For this review, take the finished solid that the model builds, in its own axes (mm). A direction names the side the tool comes from. Give positions to 0.01 mm unless a question says otherwise; leave off trailing zeros. Order: outer loops, then holes, each group sorted by start corner. A loop starts at its lowest first (then second) coordinate and runs counter-clockwise, first axis right, second up. Notation, with made-up numbers: (44.5, 35) - (103.5, 35) arc R13 cw to (103.5, 45) - close; hole circle Ø9 at (-28, -6.75). An arc over 180 degrees is marked (long way). Use a Markdown table: item, result. Add a question column.
1) Wall thickness on L1, parallel to Z at x = 4.75, y = 10.7; L2, parallel to X at y = 4.25, z = 5; L3, parallel to X at y = 5, z = 21.05: over which ranges is each line inside the solid? List them lowest first.
2) We need section A-A on x = 22.25. Write out the cut boundary in (y, z).
3) We need section D-D on z = 2. Write out the cut boundary in (x, y).
4) Mouldability with a two-part tool opening along Y and no side actions: class faces 1 (the face through (25.55, 8.41, 23.99)), 2 (the face through (2, 2, 25)), 3 (the face through (0.285, 11.699, 11.154)) as released by +Y, released by -Y, zero draft, split by the parting line, or undercut.
5) Clearance check with flat-ended pins moving along their axes: P1, Ø6.5, axis at x = 13.5, y = 5, coming from the -Z side; P2, Ø3.5, axis at x = 14.5, y = 4, coming from the +Z side; P3, Ø5.5, axis at x = 22.25, z = 8.5, coming from the -Y side; P4, Ø4, axis at x = 4.75, z = 8.5, coming from the -Y side. State where each tip first meets the part, or that it passes through.
6) We need section C-C on y = 5. Write out the cut boundary in (x, z), then the cut area to 3 significant figures.
7) We need section B-B on z = 8.5. Write out the cut boundary in (x, y).
8) Machinability: for faces 4 (the face through (25.25, 5, 10)), 5 (the face through (3.45, 8.48, 23.99)), 6 (the face through (23.55, 1.49, 23.99)), which of the approach directions +Z, -Z, +X, -X, +Y, -Y give a long, thin tool a straight path to every point of the face, cutting with its end or side? Answer none if there is none.
```python
from build123d import *

# Parameters (mm, degrees)
BOX_W           = 27
BOX_H           = 12
BOX_DEPTH       = 23
SKETCH_W        = 23.5
SKETCH_H        = 20
POCKET_DEPTH    = 10
SKETCH002_R     = 1
POCKET001_DEPTH = 3.001
SKETCH003_R     = 2
POCKET002_DEPTH = 1.5
SKETCH004_R     = 2.4
POCKET003_DEPTH = 2.001
POCKET004_DEPTH = 2.001
PAD_DEPTH       = 2
FILLET_R        = 1
FILLET001_R     = 0.8


with BuildPart() as part:
    # Box → Box (new body)
    with BuildSketch(Plane.XY):
        with Locations((13.5, 6)):
            Rectangle(BOX_W, BOX_H)
    extrude(amount=BOX_DEPTH)

    # Sketch (on Face3 of BaseFeature) → Pocket (cut)
    with BuildSketch(Plane.XZ):
        with Locations((13.5, 10)):
            Rectangle(SKETCH_W, SKETCH_H)
    extrude(amount=-POCKET_DEPTH, mode=Mode.SUBTRACT)

    # Sketch002 (on Face7 of Pocket) → Pocket001 (cut, through all)
    with BuildSketch(Plane(origin=(0, 0, 20), x_dir=(1, 0, 0), z_dir=(0, 0, -1))):
        with Locations((13.5, -5)):
            Circle(SKETCH002_R)
    extrude(amount=-POCKET001_DEPTH, mode=Mode.SUBTRACT)

    # Sketch003 (on Face7 of Pocket001) → Pocket002 (cut)
    with BuildSketch(Plane(origin=(0, 0, 20), x_dir=(1, 0, 0), z_dir=(0, 0, -1))):
        with Locations((13.5, -5)):
            Circle(SKETCH003_R)
    extrude(amount=-POCKET002_DEPTH, mode=Mode.SUBTRACT)

    # Sketch004 (on Face11 of Pocket002) → Pocket003 (cut, through all)
    with BuildSketch(Plane.XZ.offset(-10)):
        with Locations((4.75, 8.5)):
            Circle(SKETCH004_R)
        with Locations((22.25, 8.5)):
            Circle(SKETCH004_R)
    extrude(amount=-POCKET003_DEPTH, mode=Mode.SUBTRACT)

    # Sketch005 (on Face13 of Pocket003) → Pocket004 (cut, through all)
    with BuildSketch(Plane.XZ.offset(-10)):
        with BuildLine():
            ThreePointArc((16, 0), (13.5, 2.5), (11, 0))
            Line((11, 0), (16, 0))
        make_face()
    extrude(amount=-POCKET004_DEPTH, mode=Mode.SUBTRACT)

    # Sketch006 (on Face3 of Pocket004) → Pad (join)
    with BuildSketch(Plane.XY.offset(23)):
        Polygon((3.4, 9.497498), (1.402502, 9.397498), (1.502502, 7.4), (3.5, 7.5), align=None)
        Polygon((1.502502, 2.6), (3.5, 2.5), (3.4, 0.502502), (1.402502, 0.602502), align=None)
        Polygon((23.5, 2.5), (25.497498, 2.6), (25.597498, 0.602502), (23.6, 0.502502), align=None)
        Polygon((23.6, 9.497498), (25.597498, 9.397498), (25.497498, 7.4), (23.5, 7.5), align=None)
    extrude(amount=PAD_DEPTH)

    # Fillet
    fillet_edges = [part.edges().sort_by_distance(p)[0] for p in [
        (27, 6, 23),
        (27, 12, 11.5),
        (13.5, 12, 23),
        (0, 12, 11.5),
        (0, 6, 23),
    ]]
    fillet(fillet_edges, radius=FILLET_R)

    # Fillet001
    fillet001_edges = [part.edges().sort_by_distance(p)[0] for p in [
        (2.401251, 9.447498, 25),
        (2.401251, 0.552502, 25),
        (24.598749, 9.447498, 25),
        (24.598749, 0.552502, 25),
    ]]
    fillet(fillet001_edges, radius=FILLET001_R)


solid = part.part
```
Checked values:
| question | item | result |
|---|---|---|
| 1 | L1 | 0 to 6.1, 10.9 to 23 |
| 1 | L2 | 0 to 1.75, 25.25 to 27 |
| 1 | L3 | 0 to 11.5, 15.5 to 27 |
| 2 | outline | (0, 20) - (10, 20) - (10, 10.9) - (12, 10.9) - (12, 22) arc R1 ccw to (11, 23) - (0, 23) - close; (10, 0) - (12, 0) - (12, 6.1) - (10, 6.1) - close |
| 3 | outline | (0, 0) - (1.75, 0) - (1.75, 10) - (12, 10) - (12, 12) - (1, 12) arc R1 ccw to (0, 11) - close; (15, 10) - (25.25, 10) - (25.25, 0) - (27, 0) - (27, 11) arc R1 ccw to (26, 12) - (15, 12) - close |
| 4 | face 1 | undercut |
| 4 | face 2 | zero draft |
| 4 | face 3 | released by +Y |
| 5 | P1 | z = 20 |
| 5 | P2 | z = 23 |
| 5 | P3 | y = 10 |
| 5 | P4 | through |
| 6 | outline | (0, 0) - (1.75, 0) - (1.75, 20) - (11.5, 20) - (11.5, 21.5) - (12.5, 21.5) - (12.5, 23) - (1, 23) arc R1 ccw to (0, 22) - close; (14.5, 21.5) - (15.5, 21.5) - (15.5, 20) - (25.25, 20) - (25.25, 0) - (27, 0) - (27, 22) arc R1 ccw to (26, 23) - (14.5, 23) - close |
| 6 | area | 142 mm² |
| 7 | outline | (0, 0) - (1.75, 0) - (1.75, 10) - (2.35, 10) - (2.35, 12) - (1, 12) arc R1 ccw to (0, 11) - close; (7.15, 10) - (19.85, 10) - (19.85, 12) - (7.15, 12) - close; (24.65, 10) - (25.25, 10) - (25.25, 0) - (27, 0) - (27, 11) arc R1 ccw to (26, 12) - (24.65, 12) - close |
| 8 | face 4 | -Z, -Y |
| 8 | face 5 | +Z, +Y |
| 8 | face 6 | +Z, -Y |
